Check sheet for the modelled part. Datum: model origin and axes. Units: mm. Face numbers are marked on the shaded views. A direction names the side the tool comes from. Coordinates: 2 decimals unless noted, no trailing zeros. Loops run counter-clockwise (first coordinate to the right, second up) from the corner with the lowest first, then second, coordinate; pieces in that order, holes last. Notation, with made-up numbers: (86, 75) -> (95, 75) arc R20 ccw to (95, 109) -> close; hole circle Ø6 at (8.5, 13). An arc over 180 degrees is marked (long way). Use one line per item in the form item = value.
from build123d import *

# Parameters (mm, degrees)
SKETCH1_R                = 6.5
BOSS_EXTRUDE1_DEPTH      = 2
BOSS_EXTRUDE2_DEPTH      = 2
BOSS_EXTRUDE2_DEPTH_BACK = 2
BOSS_EXTRUDE3_DEPTH      = 5
BOSS_EXTRUDE3_DEPTH_BACK = 5
SKETCH3_R                = 12.5


with BuildPart() as part:
    # Sketch1 → Boss-Extrude1 (new body)
    with BuildSketch(Plane(origin=(0, 0, 0), x_dir=(1, 0, 0), z_dir=(0, 1, 0))):
        with Locations(Location((0, 0, 0), (0, 0, 270))):
            Circle(SKETCH1_R)
    extrude(amount=BOSS_EXTRUDE1_DEPTH)

    # Sketch2 → Boss-Extrude2 (add, two sides: drawn at the far end of the back side and taken through both)
    with BuildSketch(Plane.XY.offset(-BOSS_EXTRUDE2_DEPTH_BACK)):
        with BuildLine():
            Line((-2.5, 2), (-2.5, 21.005808669))
            ThreePointArc((-2.5, 21.005808669), (-0.744342007, 25.244342007), (3.494191331, 27))
            ThreePointArc((3.494191331, 27), (5.994191331, 24.5), (3.494191331, 22))
            ThreePointArc((3.494191331, 22), (2.791191899, 21.708808101), (2.5, 21.005808669))
            Line((2.5, 21.005808669), (2.5, 2))
            Line((2.5, 2), (-2.5, 2))
        make_face()
    extrude(amount=BOSS_EXTRUDE2_DEPTH + BOSS_EXTRUDE2_DEPTH_BACK)

    # Sketch3 → Boss-Extrude3 (add, two sides: drawn at the far end of the back side and taken through both)
    with BuildSketch(Plane.XY.offset(-BOSS_EXTRUDE3_DEPTH_BACK)):
        with Locations((3.494191331, 24.5)):
            Circle(SKETCH3_R)
    extrude(amount=BOSS_EXTRUDE3_DEPTH + BOSS_EXTRUDE3_DEPTH_BACK)


solid = part.part
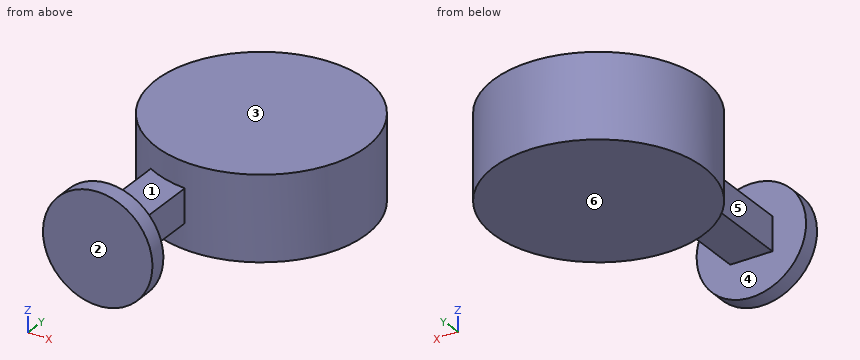
(1) Section check D-D, the plane y = 24.5. Record the boundary of the cut face in (x, z).
Established:
outline = (-9.01, -5) -> (15.99, -5) -> (15.99, 5) -> (-9.01, 5) -> close
(2) Go/stop test with flat-tipped pins: P1, Ø3, axis at y = 10.5, z = 0.5, coming from the -X side; P2, Ø1, axis at x = -1, y = 8.5, coming from the +Z side; P3, Ø4.5, axis at y = 5.5, z = 1, coming from the +X side. Record where each tip stops, or that it passes through.
Established:
P1 = -2.5
P2 = 2
P3 = 2.5
(3) Tool access check on the marked faces 5 and 6. Record the directions out of +Z, -Z, +X, -X, +Y, -Y that give a thin tool (end or side, any length) a straight path to the whole face; none if there is none.
Established:
face_5 = +Z, -Z, -X
face_6 = -Z, +X, -X, +Y
(4) Section check A-A, the plane z = 0. Record the boundary of the cut face in (x, y).
Established:
outline = (-6.5, 0) -> (6.5, 0) -> (6.5, 2) -> (2.5, 2) -> (2.5, 12.04) arc R12.5 ccw (long way) to (-2.5, 13.53) -> (-2.5, 2) -> (-6.5, 2) -> close
(5) Scan lines: line 1 along Y through (x, z) = (3.25, 3); line 2 along Z through (x, y) = (0.25, 31); line 3 along Y through (x, z) = (2.25, -2.75). Record each from-to range of solid material in increasing order.
Established:
line_1 = 0 to 2, 12 to 37
line_2 = -5 to 5
line_3 = 0 to 2, 12.06 to 36.94
(6) Section check C-C, the plane z = -3.5. Record the boundary of the cut face in (x, y), plus the area to 3 significant figures.
Established:
outline = circle Ø25 at (3.49, 24.5); (-5.48, 0) -> (5.48, 0) -> (5.48, 2) -> (-5.48, 2) -> close
area = 513 mm²
(7) Section check B-B, the plane x = -1. Record the boundary of the cut face in (y, z).
Established:
outline = (0, -6.42) -> (2, -6.42) -> (2, -2) -> (12.84, -2) -> (12.84, -5) -> (36.16, -5) -> (36.16, 5) -> (12.84, 5) -> (12.84, 2) -> (2, 2) -> (2, 6.42) -> (0, 6.42) -> close
(8) Mould release check, pull along Y, two halves, no side actions. Record for the marked faces 1, 2, 3 and 4: +Y half, -Y half, draft (parallel to the pull), parting line (faces both ways), or undercut.
Established:
face_1 = undercut
face_2 = -Y half
face_3 = draft
face_4 = undercut
